Geometry check sheet. Reference: the model listing, model coordinates, mm. Coordinates: 2 decimals unless noted, no trailing zeros. Write each loop counter-clockwise with the first axis right and the second up, starting at its lowest first coordinate (ties: lowest second). Pieces come first, ordered by that corner, then holes. Notation, with made-up numbers: (-29.75, 75.25) -> (15.25, 75.25) arc R12 ccw to (15.25, 86.25) -> close; hole circle Ø2 at (-2.75, 33). An arc over 180 degrees is marked (long way). Use a Markdown table: item, result.
```python
from build123d import *

# Parameters (mm, degrees)
ESQUISSE1_R        = 8
ESQUISSE1_R_2      = 2.25
BOSS_EXTRU_1_DEPTH = 5
BOSS_EXTRU_2_START = -5
ESQUISSE2_R        = 3
BOSS_EXTRU_2_DEPTH = 5
BOSS_EXTRU_3_START = -5
ESQUISSE3_R        = 1.5
ESQUISSE3_R_2      = 8
ESQUISSE3_R_3      = 5
BOSS_EXTRU_3_DEPTH = 5


with BuildPart() as part:
    # Esquisse1 → Boss.-Extru.1 (new body)
    with BuildSketch(Plane.XY):
        with BuildLine():
            Line((7.5, -17.5), (-7.5, -17.5))
            ThreePointArc((-7.5, -17.5), (-14.571067812, -14.571067812), (-17.5, -7.5))
            Line((-17.5, -7.5), (-17.5, 7.5))
            ThreePointArc((-17.5, 7.5), (-14.571067812, 14.571067812), (-7.5, 17.5))
            Line((-7.5, 17.5), (7.5, 17.5))
            ThreePointArc((7.5, 17.5), (14.571067812, 14.571067812), (17.5, 7.5))
            Line((17.5, 7.5), (17.5, -7.5))
            ThreePointArc((17.5, -7.5), (14.571067812, -14.571067812), (7.5, -17.5))
        make_face()
        Circle(ESQUISSE1_R, mode=Mode.SUBTRACT)
        with Locations((-10.605, 10.605)):
            Circle(ESQUISSE1_R_2, mode=Mode.SUBTRACT)
        with Locations((10.605, 10.605)):
            Circle(ESQUISSE1_R_2, mode=Mode.SUBTRACT)
        with Locations((-10.605, -10.605)):
            Circle(ESQUISSE1_R_2, mode=Mode.SUBTRACT)
        with Locations((10.605, -10.605)):
            Circle(ESQUISSE1_R_2, mode=Mode.SUBTRACT)
    extrude(amount=BOSS_EXTRU_1_DEPTH)

    # Esquisse2 → Boss.-Extru.2 (add)
    # profile 1 of 4: a face of its own
    with BuildSketch(Plane.XY.offset(5).offset(BOSS_EXTRU_2_START)):
        with BuildLine():
            Line((-37.944507823, 27.247644267), (-17.5, 6.269167951))
            Line((-17.5, 6.269167951), (-17.5, 7.5))
            ThreePointArc((-17.5, 7.5), (-14.571067812, 14.571067812), (-7.5, 17.5))
            Line((-7.5, 17.5), (-27.202072783, 37.7166504))
            ThreePointArc((-27.202072783, 37.7166504), (-30.718436651, 39.22656632), (-34.272553174, 37.807793369))
            Line((-34.272553174, 37.807793369), (-37.853364854, 34.318124658))
            ThreePointArc((-37.853364854, 34.318124658), (-39.363280773, 30.80176079), (-37.944507823, 27.247644267))
        make_face()
        with Locations((-30, 30)):
            Circle(ESQUISSE2_R, mode=Mode.SUBTRACT)
    # profile 2 of 4: a face of its own
    with BuildSketch(Plane.XY.offset(5).offset(BOSS_EXTRU_2_START)):
        with BuildLine():
            ThreePointArc((37.944507823, 27.247644267), (39.363280773, 30.80176079), (37.853364854, 34.318124658))
            Line((37.853364854, 34.318124658), (34.272553174, 37.807793369))
            ThreePointArc((34.272553174, 37.807793369), (30.718436651, 39.22656632), (27.202072783, 37.7166504))
            Line((27.202072783, 37.7166504), (7.5, 17.5))
            ThreePointArc((7.5, 17.5), (14.571067812, 14.571067812), (17.5, 7.5))
            Line((17.5, 7.5), (17.5, 6.269167951))
            Line((17.5, 6.269167951), (37.944507823, 27.247644267))
        make_face()
        with Locations((30, 30)):
            Circle(ESQUISSE2_R, mode=Mode.SUBTRACT)
    # profile 3 of 4: a face of its own
    with BuildSketch(Plane.XY.offset(5).offset(BOSS_EXTRU_2_START)):
        with BuildLine():
            Line((37.944507823, -27.247644267), (17.5, -6.269167951))
            Line((17.5, -6.269167951), (17.5, -7.5))
            ThreePointArc((17.5, -7.5), (14.571067812, -14.571067812), (7.5, -17.5))
            Line((7.5, -17.5), (27.202072783, -37.7166504))
            ThreePointArc((27.202072783, -37.7166504), (30.718436651, -39.22656632), (34.272553174, -37.807793369))
            Line((34.272553174, -37.807793369), (37.853364854, -34.318124658))
            ThreePointArc((37.853364854, -34.318124658), (39.363280773, -30.80176079), (37.944507823, -27.247644267))
        make_face()
        with Locations((30, -30)):
            Circle(ESQUISSE2_R, mode=Mode.SUBTRACT)
    # profile 4 of 4: a face of its own
    with BuildSketch(Plane.XY.offset(5).offset(BOSS_EXTRU_2_START)):
        with BuildLine():
            Line((-17.5, -7.5), (-17.5, -6.269167951))
            Line((-17.5, -6.269167951), (-37.944507823, -27.247644267))
            ThreePointArc((-37.944507823, -27.247644267), (-39.363280773, -30.80176079), (-37.853364854, -34.318124658))
            Line((-37.853364854, -34.318124658), (-34.272553174, -37.807793369))
            ThreePointArc((-34.272553174, -37.807793369), (-30.718436651, -39.22656632), (-27.202072783, -37.7166504))
            Line((-27.202072783, -37.7166504), (-7.5, -17.5))
            ThreePointArc((-7.5, -17.5), (-14.571067812, -14.571067812), (-17.5, -7.5))
        make_face()
        with Locations((-30, -30)):
            Circle(ESQUISSE2_R, mode=Mode.SUBTRACT)
    extrude(amount=BOSS_EXTRU_2_DEPTH)

    # Esquisse3 → Boss.-Extru.3 (add)
    # profile 1 of 3: a face of its own
    with BuildSketch(Plane.XY.offset(5).offset(BOSS_EXTRU_3_START)):
        Polygon((17.5, 6.269167951), (17.5, -6.269167951), (30, -19.095642241), (30, 19.095642241), align=None)
        with Locations((23, 0)):
            Circle(ESQUISSE3_R, mode=Mode.SUBTRACT)
    # profile 2 of 3: a face of its own
    with BuildSketch(Plane.XY.offset(5).offset(BOSS_EXTRU_3_START)):
        Polygon((-30, -19.095642241), (-17.5, -6.269167951), (-17.5, 6.269167951), (-30, 19.095642241), align=None)
        with Locations((-23, 0)):
            Circle(ESQUISSE3_R, mode=Mode.SUBTRACT)
    # profile 3 of 3: a face of its own
    with BuildSketch(Plane.XY.offset(5).offset(BOSS_EXTRU_3_START)):
        Circle(ESQUISSE3_R_2)
        Circle(ESQUISSE3_R_3, mode=Mode.SUBTRACT)
    extrude(amount=BOSS_EXTRU_3_DEPTH)


solid = part.part
```
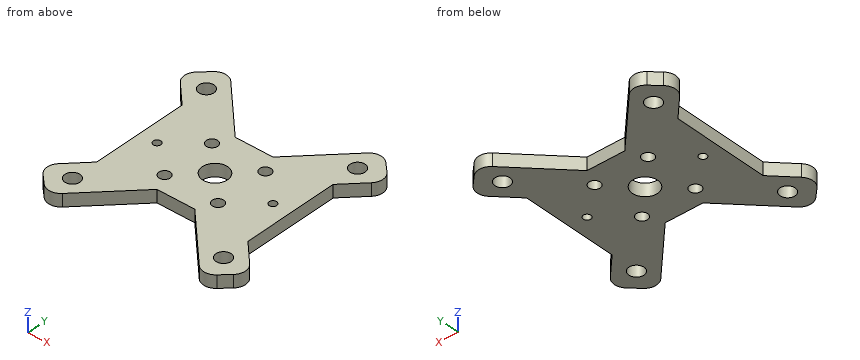
Item 1: Section check C-C on y = -24. Record the boundary of the cut face in (x, z), then the cut area to 3 significant figures.
Answer block:
| item | result |
|---|---|
| outline | (-34.78, 0) -> (-13.83, 0) -> (-13.83, 5) -> (-34.78, 5) -> close; (13.83, 0) -> (34.78, 0) -> (34.78, 5) -> (13.83, 5) -> close |
| area | 209 mm^2 |
Item 2: Section check A-A on y = 0. Record the boundary of the cut face in (x, z).
Answer block:
| item | result |
|---|---|
| outline | (-30, 0) -> (-24.5, 0) -> (-24.5, 5) -> (-30, 5) -> close; (-21.5, 0) -> (-5, 0) -> (-5, 5) -> (-21.5, 5) -> close; (5, 0) -> (21.5, 0) -> (21.5, 5) -> (5, 5) -> close; (24.5, 0) -> (30, 0) -> (30, 5) -> (24.5, 5) -> close |
Item 3: Section check D-D on x = 29. Record the boundary of the cut face in (y, z), then the cut area to 3 significant figures.
Answer block:
| item | result |
|---|---|
| outline | (-38.9, 0) -> (-32.83, 0) -> (-32.83, 5) -> (-38.9, 5) -> close; (-27.17, 0) -> (27.17, 0) -> (27.17, 5) -> (-27.17, 5) -> close; (32.83, 0) -> (38.9, 0) -> (38.9, 5) -> (32.83, 5) -> close |
| area | 332 mm^2 |
Item 4: Depth check by flat-ended pin: P1, Ø1.5, axis at y = -2.5, z = 3, coming from the -X side; P2, Ø2, axis at x = 14.5, z = 1.5, coming from the +Y side; P3, Ø1.5, axis at x = 24, y = -13.5, coming from the -Z side; P4, Ø2.5, axis at x = -0.5, z = 3.5, coming from the -Y side. Enter the tip coordinate at first touch or a pass-through.
Answer block:
| item | result |
|---|---|
| P1 | stops at x = -30 |
| P2 | stops at y = 25.71 |
| P3 | stops at z = 0 |
| P4 | stops at y = -17.5 |
Item 5: Thickness scan on L1, parallel to Y at x = 0, z = 3.3; L2, parallel to X at y = -14, z = 2.45; L3, parallel to Y at x = -10, z = 2.75. Record the ranges inside material, lowest first. Write a range as [from, to].
Answer block:
| item | result |
|---|---|
| L1 | y = [-17.5, -5], [5, 17.5] |
| L2 | x = [-30, 30] |
| L3 | y = [-20.07, -12.77], [-8.44, 8.44], [12.77, 20.07] |
Item 6: Section check B-B on x = -23. Record the boundary of the cut face in (y, z).
Answer block:
| item | result |
|---|---|
| outline | (-33.4, 0) -> (-1.5, 0) -> (-1.5, 5) -> (-33.4, 5) -> close; (1.5, 0) -> (33.4, 0) -> (33.4, 5) -> (1.5, 5) -> close |
